```python
from build123d import *

# Parameters (mm, degrees)
SKETCH4_R           = 2.25
SKETCH4_R_2         = 7.9375
BOSS_EXTRUDE1_DEPTH = 5
CUT_EXTRUDE1_DEPTH  = 191.5


with BuildPart() as part:
    # Sketch4 → Boss-Extrude1 (new body)
    with BuildSketch(Plane.XY):
        with BuildLine():
            Line((-66.080112923, -1201.56262), (96.419887077, -1201.56262))
            ThreePointArc((96.419887077, -1201.56262), (106.319382013, -1197.462114937), (110.419887077, -1187.56262))
            Line((110.419887077, -1187.56262), (110.419887077, -812.43738))
            ThreePointArc((110.419887077, -812.43738), (106.319382013, -802.537885063), (96.419887077, -798.43738))
            Line((96.419887077, -798.43738), (-66.080112923, -798.43738))
            ThreePointArc((-66.080112923, -798.43738), (-75.97960786, -802.537885063), (-80.080112923, -812.43738))
            Line((-80.080112923, -812.43738), (-80.080112923, -1187.56262))
            ThreePointArc((-80.080112923, -1187.56262), (-75.97960786, -1197.462114937), (-66.080112923, -1201.56262))
        make_face()
        with Locations((96.419887077, -1080)):
            Circle(SKETCH4_R, mode=Mode.SUBTRACT)
        with Locations((88.147808187, -1029.0799835)):
            Circle(SKETCH4_R_2, mode=Mode.SUBTRACT)
        with Locations((-66.080112923, -1080)):
            Circle(SKETCH4_R, mode=Mode.SUBTRACT)
        with Locations((96.419887077, -920)):
            Circle(SKETCH4_R, mode=Mode.SUBTRACT)
        with Locations((-66.080112923, -920)):
            Circle(SKETCH4_R, mode=Mode.SUBTRACT)
        with Locations((-66.080112923, -1187.56262)):
            Circle(SKETCH4_R, mode=Mode.SUBTRACT)
        with Locations((96.419887077, -1187.56262)):
            Circle(SKETCH4_R, mode=Mode.SUBTRACT)
        with Locations((-66.080112923, -812.43738)):
            Circle(SKETCH4_R, mode=Mode.SUBTRACT)
        with Locations((96.419887077, -812.43738)):
            Circle(SKETCH4_R, mode=Mode.SUBTRACT)
    extrude(amount=BOSS_EXTRUDE1_DEPTH)

    # Sketch6 → Cut-Extrude1 (cut, through all)
    with BuildSketch(Plane(origin=(110.419887077, 0, 0), x_dir=(0, 0, -1), z_dir=(1, 0, 0))):
        Polygon((-5, -990), (-2.5, -990), (-2.5, -1000), (0, -1000), (102.688211321, -812.43738), (-56.641520251, -690.463913443), (-113.62806658, -898.225606144), align=None)
    extrude(amount=-CUT_EXTRUDE1_DEPTH, mode=Mode.SUBTRACT)


solid = part.part
```
CAD build for the part. Positions are in the model's coordinates, mm. A direction names the side the tool comes from. Coordinates: 2 decimals unless noted, no trailing zeros. Loops run counter-clockwise (first coordinate to the right, second up) from the corner with the lowest first, then second, coordinate; pieces in that order, holes last. Notation, with made-up numbers: (-4, 46) - (46, 46) arc R32 ccw to (46, 73) - close; hole circle Ø2 at (84.5, -37.75). An arc over 180 degrees is marked (long way). Return JSON: item names as keys, results as strings.
1. Band-saw the part on A-A (x = -7.5). Give the cut face in (y, z).
Result:
{"outline": "(-1201.56, 0) - (-1000, 0) - (-1000, 2.5) - (-990, 2.5) - (-990, 5) - (-1201.56, 5) - close"}
2. 3-axis set-ups, long thin cutter, end or side, ignore diameter. For faces 4 (the flat face through (14, -1201.563, 2)), 5 (the flat face through (17, -995, 2.5)): which of +Z, -Z, +X, -X, +Y, -Y reach the whole face in a straight line?
Result:
{"face 4": "+Z, -Z, +X, -X, -Y", "face 5": "-Z, +X, -X, +Y"}
3. Mould opens along X. For faces 1 (the flat face through (14, -1099, 0)), 2 (the cylindrical face through (-66.568, -1082.196, 2.465)), 3 (the flat face through (-80.08, -1087, 2)) say: released by +X, released by -X, zero draft, split by the parting line, or undercut.
Result:
{"face 1": "zero draft", "face 2": "undercut", "face 3": "released by -X"}
4. Drop flat-ended pins along their axis: pin 1 (1.5 mm diameter, centred on x = 4, z = 1, fed in from +Y); pin 2 (8 mm diameter, centred on x = 41, y = -993.5, fed in from -Z). Give the stop position or say it passes through.
Result:
{"pin 1": "stops at y = -1000", "pin 2": "stops at z = 2.5"}
5. Probe L1, parallel to X at y = -1080, z = 1.05; L2, parallel to Y at x = 89.5, z = 0.9; L3, parallel to Y at x = -55.5, z = 2.4. List the from-to ranges inside material, lowest first. Write a range as from..to.
Result:
{"L1": "x = -80.08..-68.33, -63.83..94.17, 98.67..110.42", "L2": "y = -1201.56..-1036.9, -1021.26..-1000", "L3": "y = -1201.56..-1000"}
